```python
from build123d import *

# Parameters (mm, degrees)
SKETCH_1_R                = 20
SKETCH_1_R_2              = 11.1
EXTRUDE_1_DEPTH           = 60
EXTRUDE_2_DEPTH           = 30
SKETCH_4_R                = 11
EXTRUDE_3_DEPTH           = 5
SKETCH_8_R                = 11.1
CUT_EXTRUDE_1_DEPTH       = 100
FILLET_4_R                = 20
EXTRUDE_START             = -30
SKETCH_18_R               = 35
EXTRUDE_4_DEPTH           = 5
EXTRUDE_START_2           = -25
SKETCH_19_R               = 35
EXTRUDE_5_DEPTH           = 5
FILLET_5_R                = 10
CUT_EXTRUDE_9_DEPTH       = 388.169213652
CUT_EXTRUDE_9_DEPTH_BACK  = 388.169213652
SKETCH_21_R               = 2.6
CUT_EXTRUDE_10_DEPTH      = 407.881000043
CUT_EXTRUDE_10_DEPTH_BACK = 407.881000043
SKETCH_22_W               = 45
SKETCH_22_H               = 451.378457943
SKETCH_22_W_2             = 20
SKETCH_22_H_2             = 431.087956996


with BuildPart() as part:
    # 草图1 → 凸台-拉伸1 (new body)
    with BuildSketch(Plane.XY):
        Circle(SKETCH_1_R)
        Circle(SKETCH_1_R_2, mode=Mode.SUBTRACT)
    extrude(amount=EXTRUDE_1_DEPTH)

    # 草图2 → 凸台-拉伸2 (add, symmetric)
    with BuildSketch(Plane.XY.offset(30)):
        with BuildLine():
            Line((-14.142135624, 14.142135624), (-90, -61.715728753))
            Line((-90, -61.715728753), (-90, -320))
            Line((-90, -320), (-50, -320))
            Line((-50, -320), (-50, -78.284271247))
            Line((-50, -78.284271247), (14.142135624, -14.142135624))
            ThreePointArc((14.142135624, -14.142135624), (-14.142135624, -14.142135624), (-14.142135624, 14.142135624))
        make_face()
    extrude(amount=EXTRUDE_2_DEPTH, both=True)

    # 草图4 → 凸台-拉伸3 (add)
    with BuildSketch(Plane.XY.offset(60)):
        with BuildLine():
            Line((-90, -290), (-50, -290))
            Line((-50, -290), (-50, -350))
            ThreePointArc((-50, -350), (-70, -370), (-90, -350))
            Line((-90, -350), (-90, -290))
        make_face()
        with Locations((-70, -350)):
            Circle(SKETCH_4_R, mode=Mode.SUBTRACT)
    extrude_3 = extrude(amount=EXTRUDE_3_DEPTH)

    # 镜向1: 凸台-拉伸3 across plane
    add(extrude_3.mirror(Plane.XY.offset(30)))

    # 草图8 → 切除-拉伸1 (cut)
    with BuildSketch(Plane.XY.offset(60)):
        with Locations((-35.355339059, -35.355339059)):
            Circle(SKETCH_8_R)
    extrude(amount=-CUT_EXTRUDE_1_DEPTH, mode=Mode.SUBTRACT)

    # 圆角4
    fillet_4_edges = [part.edges().sort_by_distance(p)[0] for p in [
        (-50, -78.284271247, 30),
        (-90, -61.715728753, 30),
    ]]
    fillet(fillet_4_edges, radius=FILLET_4_R)

    # 草图18 → 凸台-拉伸4 (add)
    with BuildSketch(Plane.XY.offset(60).offset(EXTRUDE_START)):
        with BuildLine():
            ThreePointArc((15.487252676, -12.654841151), (14.833346688, -13.415357842), (14.142135624, -14.142135624))
            Line((14.142135624, -14.142135624), (-44.142135624, -72.426406871))
            ThreePointArc((-44.142135624, -72.426406871), (-48.47759065, -78.914873848), (-50, -86.568542495))
            Line((-50, -86.568542495), (-50, -128.513280962))
            Line((-50, -128.513280962), (20.291868618, -128.513280962))
            ThreePointArc((20.291868618, -128.513280962), (62.790327113, -100.116718851), (52.818780552, -49.986369028))
            Line((52.818780552, -49.986369028), (15.487252676, -12.654841151))
        make_face()
        with Locations((20.291868618, -82.513280962)):
            Circle(SKETCH_18_R, mode=Mode.SUBTRACT)
    extrude(amount=EXTRUDE_4_DEPTH)

    # 草图19 → 凸台-拉伸5 (add)
    with BuildSketch(Plane(origin=(0, 0, 0), x_dir=(-1, 0, 0), z_dir=(0, 0, -1)).offset(EXTRUDE_START_2)):
        with BuildLine():
            Line((50, -134.571348531), (50, -226.571348531))
            Line((50, -226.571348531), (-0.680255104, -226.571348531))
            ThreePointArc((-0.680255104, -226.571348531), (-46.680255104, -180.571348531), (-0.680255104, -134.571348531))
            Line((-0.680255104, -134.571348531), (50, -134.571348531))
        make_face()
        with Locations((-0.680255104, -180.571348531)):
            Circle(SKETCH_19_R, mode=Mode.SUBTRACT)
    extrude(amount=-EXTRUDE_5_DEPTH)

    # 圆角5
    # the kernel refuses this fillet: 10 mm, written as the material it adds along each edge
    with BuildSketch(Plane(origin=(-50, -226.571348531, 25), x_dir=(0, -1, 0), z_dir=(0, 0, 1)), Plane(origin=(-50, -128.513280962, 30), x_dir=(0, -1, 0), z_dir=(0, 0, 1))) as fillet_5_piece_1:
        with BuildLine():
            CenterArc((FILLET_5_R, FILLET_5_R), FILLET_5_R, 180, 90)
            Line((0, FILLET_5_R), (0, 0))
            Line((0, 0), (FILLET_5_R, 0))
        make_face()
    extrude(amount=5)

    # 草图21 → 切除-拉伸9 (cut, two sides: drawn at the far end of the back side and taken through both)
    with BuildSketch(Plane.XY.offset(65).offset(-CUT_EXTRUDE_9_DEPTH_BACK)):
        with Locations((-70, -75)):
            Circle(SKETCH_21_R)
        with Locations((-70, -250)):
            Circle(SKETCH_21_R)
        with Locations((-58, -300)):
            Circle(SKETCH_21_R)
        with Locations((-82, -300)):
            Circle(SKETCH_21_R)
    extrude(amount=CUT_EXTRUDE_9_DEPTH + CUT_EXTRUDE_9_DEPTH_BACK, mode=Mode.SUBTRACT)

    # 草图22 → 切除-拉伸10 (cut, two sides: drawn at the far end of the back side and taken through both)
    with BuildSketch(Plane.ZY.offset(90).offset(-CUT_EXTRUDE_10_DEPTH_BACK)):
        with Locations((17.5, -160.771309387)):
            Rectangle(SKETCH_22_W, SKETCH_22_H)
        with Locations((55, -154.456021502)):
            Rectangle(SKETCH_22_W_2, SKETCH_22_H_2)
    extrude(amount=CUT_EXTRUDE_10_DEPTH + CUT_EXTRUDE_10_DEPTH_BACK, mode=Mode.SUBTRACT)


solid = part.part
```
The model under review builds one solid part; all positions refer to its coordinate system, in mm. Give positions to 0.01 mm unless a question says otherwise; leave off trailing zeros. Write each loop counter-clockwise with the first axis right and the second up, starting at its lowest first coordinate (ties: lowest second). Pieces come first, ordered by that corner, then holes. Notation, with made-up numbers: M 15,38 L 55,38 A19 cw 55,71 Z; hole C -9,40 d10. An arc over 180 degrees is marked long. Write item = value, one per line. Start each with the question number.
Q1. For line 1 (X direction, y = -300, z = 42.7); line 2 (Y direction, x = -68, z = 43.6); line 3 (X direction, y = -173, z = 43.7), list the stretches that pass through material, from the lowest coordinate up.
Q2. We need section A-A (x = 0). State the section outline as (y, z) points, plus the area to 3 significant figures.
Q3. We need section D-D (x = -41). State the section outline as (y, z) points.
Q4. We need section B-B (z = 42). State the section outline as (x, y) points.
Q5. Clearance check with flat-ended pins moving along their axes: pin 1 (4 mm diameter, centred on x = -82, y = -300, fed in from -Z); pin 2 (1.5 mm diameter, centred on y = -154.5, z = 42, fed in from +X). State where each tip first meets the part, or that it passes through.
Q6. We need section C-C (y = -181). State the section outline as (x, z) points.
Q7. Mouldability with a two-part tool opening along Y and no side actions: class faces 1 (the face through (-59, -151, 40)), 2 (the face through (-48.52, -79.02, 42.46)), 3 (the face through (5.97, 9.36, 42.46)) as released by +Y, released by -Y, zero draft, split by the parting line, or undercut.
Result set:
q1.line_1 = -90 to -84.6, -79.4 to -60.6, -55.4 to -50
q1.line_2 = -320 to -251.66, -248.34 to -76.66, -73.34 to -39.72
q1.line_3 = -90 to -50
q2.outline = M -28.28,40 L -11.1,40 L -11.1,45 L -28.28,45 Z; M 11.1,40 L 20,40 L 20,45 L 11.1,45 Z
q2.area = 130 mm2
q3.outline = M -69.28,40 L -44.91,40 L -44.91,45 L -69.28,45 Z; M -25.8,40 L -12.72,40 L -12.72,45 L -25.8,45 Z
q4.outline = M -90,-320 L -50,-320 L -50,-86.57 A20 cw -44.14,-72.43 L 14.14,-14.14 A20 ccw -14.14,14.14 L -84.14,-55.86 A20 ccw -90,-70 Z; hole C -82,-300 d5.2; hole C -70,-250 d5.2; hole C -70,-75 d5.2; hole C -58,-300 d5.2; hole C -35.36,-35.36 d22.2; hole C 0,0 d22.2
q5.pin_1 = through
q5.pin_2 = -50
q6.outline = M -90,40 L -50,40 L -50,45 L -90,45 Z
q7.face_1 = zero draft
q7.face_2 = released by -Y
q7.face_3 = undercut
